Source: CAD feature listing. Evaluate the final solid. Frame: model axes, mm. A direction names the side the tool comes from. Round coordinates to 2 decimals unless told otherwise and drop trailing zeros. Order: outer loops, then holes, each group sorted by start corner. A loop starts at its lowest first (then second) coordinate and runs counter-clockwise, first axis right, second up. Notation, with made-up numbers: M -36.5,-18 L -1.5,-18 A17 cw -1.5,0 Z; hole C 36,19.25 d9. An arc over 180 degrees is marked long. Answer as CSV lines item,"result". Start each with the question number.
Item 1: Pull-direction query (Y, two-part tool) for faces 1 (the face through (12, 0, 38)), 2 (the face through (19, -15, 10)), 3 (the face through (6, -15, 10)), 4 (the face through (25, -10, 38)); classes: +Y half, -Y half, draft (parallel to the pull), parting line (faces both ways), or undercut.
Item 2: Section query A-A on x = 12.5. Return the cut outline in (y, z), plus the area to 3 significant figures.
Item 3: Line query: line 1 (Y direction, x = 12.5, z = 5.25); line 2 (Y direction, x = 18.75, z = 71.75). Output: solid intervals per line, ascending. Write a range as [from, to].
Item 4: Set-up query: faces 5 (the face through (5.536, -16.373, 4.93)), 6 (the face through (0, -10, 38)), 7 (the face through (17.25, -14.93, 73.07)). Return all of +Z, -Z, +X, -X, +Y, -Y with unobstructed straight access to the full face (end or side cutting, diameter ignored); none if empty.
Item 5: Section query B-B on y = -5. Return the cut outline in (x, z).
Item 6: First-contact query: P1, Ø2.5, axis at x = 6.25, y = -15, coming from the -Z side; P2, Ø0.9, axis at x = 19.5, y = -14.5, coming from the +Z side. Flat tips, straight axial feed; report the tip coordinate or a pass-through.
from build123d import *

# Parameters (mm, degrees)
SKETCH1_W           = 25
SKETCH1_H           = 20
BOSS_EXTRUDE2_DEPTH = 78
SKETCH3_R           = 1.5
CUT_EXTRUDE2_DEPTH  = 10
SKETCH6_R           = 1.485523147
SKETCH6_R_2         = 1.547360616
SKETCH6_R_3         = 1.494600316
CUT_EXTRUDE3_DEPTH  = 10


with BuildPart() as part:
    # Sketch1 → Boss-Extrude2 (new body)
    with BuildSketch(Plane.XY):
        with Locations((12.5, -10)):
            Rectangle(SKETCH1_W, SKETCH1_H)
    extrude(amount=BOSS_EXTRUDE2_DEPTH)

    # Sketch3 → Cut-Extrude2 (cut)
    with BuildSketch(Plane.XY.offset(78)):
        with Locations((6.25, -15)):
            Circle(SKETCH3_R)
        with Locations((12.5, -5)):
            Circle(SKETCH3_R)
        with Locations((18.75, -15)):
            Circle(SKETCH3_R)
    extrude(amount=-CUT_EXTRUDE2_DEPTH, mode=Mode.SUBTRACT)

    # Sketch6 → Cut-Extrude3 (cut)
    with BuildSketch(Plane(origin=(0, 0, 0), x_dir=(-1, 0, 0), z_dir=(0, 0, -1))):
        with Locations((-12.5, -5)):
            Circle(SKETCH6_R)
        with Locations((-6.25, -15)):
            Circle(SKETCH6_R_2)
        with Locations((-18.75, -15)):
            Circle(SKETCH6_R_3)
    extrude(amount=-CUT_EXTRUDE3_DEPTH, mode=Mode.SUBTRACT)


solid = part.part
Results:
1,face 1,"+Y half"
1,face 2,"undercut"
1,face 3,"undercut"
1,face 4,"draft"
2,outline,"M -20,0 L -6.49,0 L -6.49,10 L -3.51,10 L -3.51,0 L 0,0 L 0,78 L -3.5,78 L -3.5,68 L -6.5,68 L -6.5,78 L -20,78 Z"
2,area,"1,500 mm^2"
3,line 1,"[-20, -6.49], [-3.51, 0]"
3,line 2,"[-20, -16.5], [-13.5, 0]"
4,face 5,"-Z"
4,face 6,"+Z, -Z, -X, +Y, -Y"
4,face 7,"+Z"
5,outline,"M 0,0 L 11.01,0 L 11.01,10 L 13.99,10 L 13.99,0 L 25,0 L 25,78 L 14,78 L 14,68 L 11,68 L 11,78 L 0,78 Z"
6,P1,"z = 10"
6,P2,"z = 68"
